Read the model definition and answer for the solid it produces. Units are mm, in the model's axes. A direction names the side the tool comes from. Coordinates: 2 decimals unless noted, no trailing zeros. Order: outer loops, then holes, each group sorted by start corner. A loop starts at its lowest first (then second) coordinate and runs counter-clockwise, first axis right, second up. Notation, with made-up numbers: (29.25, 84.5) - (35.25, 84.5) arc R8 ccw to (35.25, 94.5) - close; hole circle Ø11 at (27.5, 79.25). An arc over 180 degrees is marked (long way). Write item = value, one per line.
from build123d import *

# Parameters (mm, degrees)
BOSS_EXTRUDE1_DEPTH = 1.25
BOSS_EXTRUDE2_DEPTH = 9.5
CHAMFER1_SIZE       = 5
FILLET1_R           = 5


with BuildPart() as part:
    # Sketch1 → Boss-Extrude1 (new, symmetric)
    with BuildSketch(Plane.XY):
        with BuildLine():
            Line((0, 0), (0, -45))
            ThreePointArc((0, -45), (-36.286223281, -43.748513109), (-72.4, -40))
            ThreePointArc((-72.4, -40), (-114.06327772, -29.435407254), (-152.4, -10))
            ThreePointArc((-152.4, -10), (-117.755339059, -2.512626585), (-82.4, 0))
            Line((-82.4, 0), (0, 0))
        make_face()
    extrude(amount=BOSS_EXTRUDE1_DEPTH, both=True)

    # Sketch2 → Boss-Extrude2 (add, symmetric)
    with BuildSketch(Plane.XY):
        with BuildLine():
            Line((0, 0), (128, 0))
            ThreePointArc((128, 0), (134.5, -1.3), (140, -5))
            ThreePointArc((140, -5), (141.968086361, -18.167413874), (130, -24))
            ThreePointArc((130, -24), (122.876979683, -20.60373569), (114.994710808, -20.227083248))
            ThreePointArc((114.994710808, -20.227083248), (69.989649226, -23.594360459), (24.994710808, -20.094411808))
            ThreePointArc((24.994710808, -20.094411808), (24.383812263, -20.023637874), (23.769282172, -20))
            Line((23.769282172, -20), (18.769282172, -20))
            ThreePointArc((18.769282172, -20), (17.12660254, -20.557614597), (16.162831426, -22))
            Line((16.162831426, -22), (10, -45))
            Line((10, -45), (0, -45))
            Line((0, -45), (0, 0))
        make_face()
    extrude(amount=BOSS_EXTRUDE2_DEPTH, both=True)

    # Chamfer1
    chamfer1_edges = [part.edges().sort_by_distance(p)[0] for p in [
        (0, -22.5, -9.5),
        (0, -22.5, 9.5),
    ]]
    chamfer(chamfer1_edges, length=CHAMFER1_SIZE)

    # Fillet1
    fillet1_edges = [part.edges().sort_by_distance(p)[0] for p in [
        (13.081415713, -33.5, -9.5),
        (17.12660254, -20.557614597, -9.5),
        (21.269282172, -20, -9.5),
        (24.383812263, -20.023637874, -9.5),
        (122.876979683, -20.60373569, -9.5),
        (141.968086361, -18.167413874, -9.5),
        (134.5, -1.3, -9.5),
        (13.081415713, -33.5, 9.5),
        (17.12660254, -20.557614597, 9.5),
        (21.269282172, -20, 9.5),
        (24.383812263, -20.023637874, 9.5),
        (122.876979683, -20.60373569, 9.5),
        (141.968086361, -18.167413874, 9.5),
        (134.5, -1.3, 9.5),
        (69.989649226, -23.594360459, -9.5),
        (66.5, 0, -9.5),
        (69.989649226, -23.594360459, 9.5),
        (66.5, 0, 9.5),
    ]]
    fillet(fillet1_edges, radius=FILLET1_R)


solid = part.part
1) The part is cut by section A-A (x = -34). Determine the outline of the cut face in (y, z), and give its area (3 significant figures).
Returned:
outline = (-43.9, -1.25) - (0, -1.25) - (0, 1.25) - (-43.9, 1.25) - close
area = 110 mm^2
2) For faces 1 (the face through (21.23, -18.5, 8.07)), 2 (the face through (-58, -17, -1.25)), 3 (the face through (-58, -17, 1.25)), 4 (the face through (21, -20, 0)), 5 (the face through (134.414, -1.264, 0.063)), determine the directions among +Z, -Z, +X, -X, +Y, -Y from which every point of the face is accessible in a straight line to the end or side of a thin tool.
Returned:
face_1 = +Z, -Y
face_2 = -Z, -X, +Y, -Y
face_3 = +Z, -X, +Y, -Y
face_4 = +Z, -Z, -Y
face_5 = +Z, -Z, +X, +Y
3) The part is cut by section B-B (x = -119.5). Determine the outline of the cut face in (y, z).
Returned:
outline = (-27.3, -1.25) - (-2.77, -1.25) - (-2.77, 1.25) - (-27.3, 1.25) - close
4) Straight lines are drawn through the part: line 1 along Z through (x, y) = (-76, -12); line 2 along X through (y, z) = (-41, 4.75); line 3 along X through (y, z) = (-39, 8.5). For each, find the intervals that lie inside material, in ascending order. Write a range as from..to.
Returned:
line_1 = -1.25..1.25
line_2 = 0.25..11.07
line_3 = 4..9.54
5) Flat-ended cylindrical pins translate along their axes: pin 1 Ø5 at (x, y) = (-56, -4.5) entering from -Z; pin 2 Ø1 at (y, z) = (-23.5, -2) entering from -X; pin 3 Ø22.5 at (x, y) = (-80, -17.5) entering from +Z. Find the tip coordinate at first contact, or state that the pin passes through.
Returned:
pin_1 = -1.25
pin_2 = 0
pin_3 = 1.25
